Answer from the drawing. Dimensions are ordinates in mm from the lowest x, y and z of the part. A direction names the side the tool comes from. Coordinates: 2 decimals unless noted, no trailing zeros. Write each loop counter-clockwise with the first axis right and the second up, starting at its lowest first coordinate (ties: lowest second). Pieces come first, ordered by that corner, then holes. Notation, with made-up numbers: M 0,37.25 L 10,37.25 A21 ccw 10,59.25 Z; hole C 12,-11 d3. An arc over 180 degrees is marked long. Put each result on its own line as item: value. Start each with the question number.
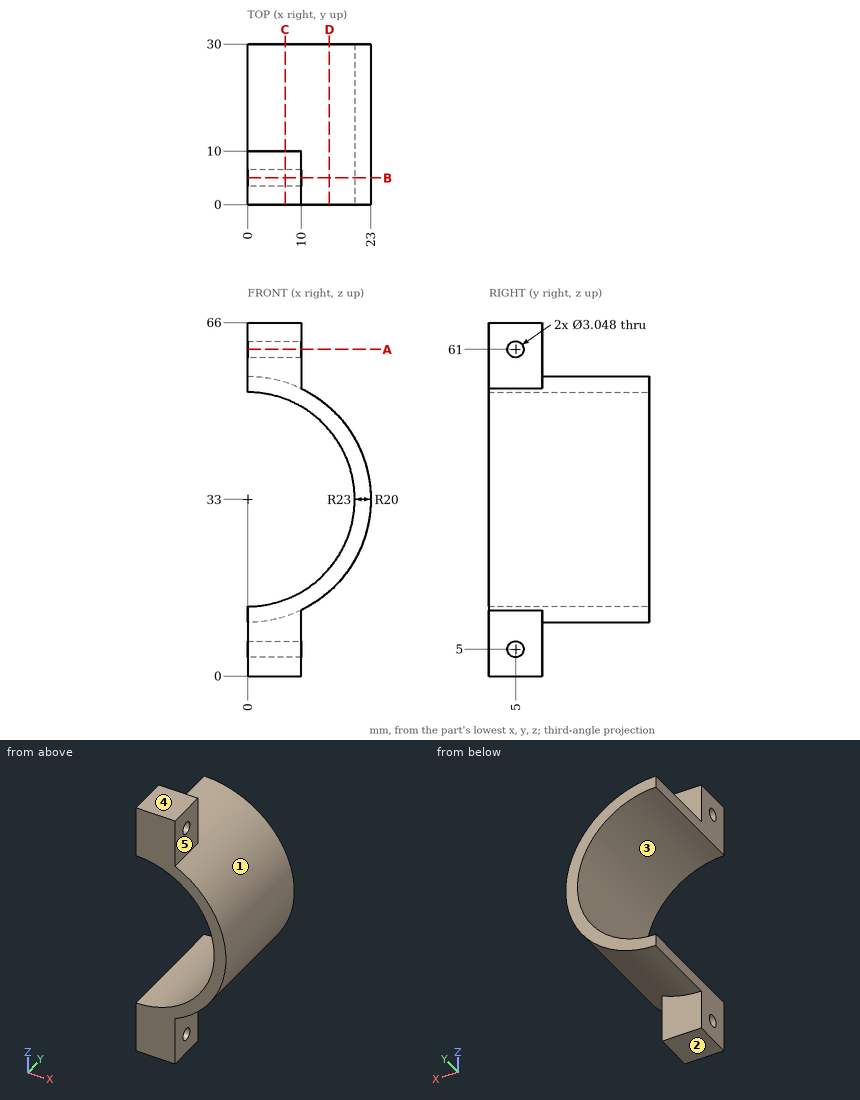
1) Straight lines are drawn through the part: probe 1 along Y at (x, z) = (6.75, 5); probe 2 along Z at (x, y) = (18.5, 26.5); probe 3 along X at (y, z) = (2, 9). For each, find the intervals that lie inside material, in ascending order.
2) Determine the mould class of the marked faces 3, 4 and 5 for opening direction Z: +Z half, -Z half, draft (parallel to the pull), parting line (faces both ways), or undercut.
3) A cutting plane is placed at A-A on z = 61. Write down the section's boundary in (x, y), then the cut area to 3 significant figures.
4) A cutting plane is placed at C-C on x = 7. Write down the section's boundary in (y, z) (3 decimals), then the cut area to 3 significant figures.
5) Given pin 1 Ø5 at (y, z) = (6.5, 5.5) entering from +X; pin 2 Ø8 at (x, y) = (4, 16) entering from -Z; pin 3 Ø8 at (x, z) = (7.5, 6.5) entering from +Y, each flat-ended and moving along its own axis, determine where each tip first touches the part or whether it passes through.
6) For the marked faces 1 and 2, determine the directions among +Z, -Z, +X, -X, +Y, -Y from which every point of the face is accessible in a straight line to the end or side of a thin tool.
7) A cutting plane is placed at D-D on x = 15.25. Write down the section's boundary in (y, z).
8) A cutting plane is placed at B-B on y = 5. Write down the section's boundary in (x, z).
Answers follow:
1. probe 1: y = 0 to 3.48, 6.52 to 10
1. probe 2: z = 19.33 to 25.4, 40.6 to 46.67
1. probe 3: x = 0 to 10
2. face 3: undercut
2. face 4: +Z half
2. face 5: draft
3. outline: M 0,0 L 10,0 L 10,3.48 L 0,3.48 Z; M 0,6.52 L 10,6.52 L 10,10 L 0,10 Z
3. area: 69.5 mm²
4. outline: M 0,0 L 10,0 L 10,11.091 L 30,11.091 L 30,14.265 L 0,14.265 Z; M 0,51.735 L 30,51.735 L 30,54.909 L 10,54.909 L 10,66 L 0,66 Z; hole C 5,5 d3.048; hole C 5,61 d3.048
4. area: 398 mm²
5. pin 1: stops at x = 10
5. pin 2: stops at z = 10
5. pin 3: stops at y = 10
6. face 1: +X, +Y
6. face 2: -Z, +X, -X, +Y, -Y
7. outline: M 0,15.78 L 30,15.78 L 30,20.06 L 0,20.06 Z; M 0,45.94 L 30,45.94 L 30,50.22 L 0,50.22 Z
8. outline: M 0,0 L 10,0 L 10,3.48 L 0,3.48 Z; M 0,6.52 L 10,6.52 L 10,12.29 A23 ccw 10,53.71 L 10,59.48 L 0,59.48 L 0,53 A20 cw 0,13 Z; M 0,62.52 L 10,62.52 L 10,66 L 0,66 Z
